from build123d import *

# Parameters (mm, degrees)
SKETCH3_R          = 4
CUT_EXTRUDE1_DEPTH = 14


with BuildPart() as part:
    # Sketch2 → Revolve1 (revolve)
    with BuildSketch(Plane(origin=(0, 0, 0), x_dir=(0, 0, -1), z_dir=(1, 0, 0)), mode=Mode.PRIVATE) as revolve1_sk:
        with BuildLine():
            Line((68.94, 0), (68.94, 32))
            Line((68.94, 32), (80, 32))
            Line((80, 32), (89.743935399, 25.177222982))
            ThreePointArc((89.743935399, 25.177222982), (86.850368108, 16), (89.743935399, 6.822777018))
            Line((89.743935399, 6.822777018), (80, 0))
            Line((80, 0), (68.94, 0))
        make_face()
    revolve(revolve1_sk.sketch.rotate(Axis((0, 24.773264932, 0), (0, -1, 0)), 180), axis=Axis((0, 24.773264932, 0), (0, -1, 0)))

    # Sketch3 → Cut-Extrude1 (cut)
    with BuildSketch(Plane(origin=(0, 0, 0), x_dir=(1, 0, 0), z_dir=(0, 1, 0))):
        with Locations((0, 68.94)):
            Circle(SKETCH3_R)
        with Locations((48.747941495, 48.747941495)):
            Circle(SKETCH3_R)
        with Locations((68.94, 0)):
            Circle(SKETCH3_R)
        with Locations((48.747941495, -48.747941495)):
            Circle(SKETCH3_R)
        with Locations((0, -68.94)):
            Circle(SKETCH3_R)
        with Locations((-48.747941495, -48.747941495)):
            Circle(SKETCH3_R)
        with Locations((-68.94, 0)):
            Circle(SKETCH3_R)
        with Locations((-48.747941495, 48.747941495)):
            Circle(SKETCH3_R)
    extrude(amount=CUT_EXTRUDE1_DEPTH, mode=Mode.SUBTRACT)


solid = part.part
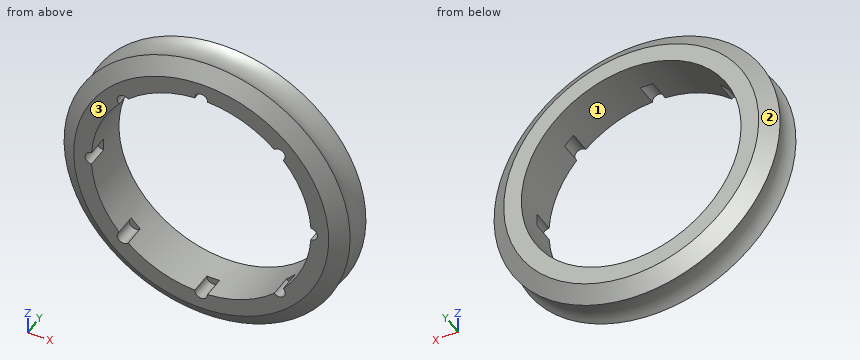
Verification items for the finished model (mm, model axes). Face numbers are marked on the shaded views. Round coordinates to 2 decimals unless told otherwise and drop trailing zeros. Loops run counter-clockwise (first coordinate to the right, second up) from the corner with the lowest first, then second, coordinate; pieces in that order, holes last. Notation, with made-up numbers: M 58.25,-19.5 L 88.25,-19.5 A15 cw 88.25,2.5 Z; hole C 81.5,75 d5. An arc over 180 degrees is marked long. Write each question's results on one line, items separated by ' | '.
1) Section check D-D on y = 17. Record the boundary of the cut face in (x, z).
Checks:
outline: C 0,0 d173.76; hole C 0,0 d137.88
2) Section check C-C on y = 28.5. Record the boundary of the cut face in (x, z).
Checks:
outline: C 0,0 d170; hole C 0,0 d137.88
3) Scan lines: L1, parallel to X at y = 15, z = 30.5; L2, parallel to X at y = 11, z = -62; L3, parallel to Z at x = -14.5, y = 6.5. Record each from-to range of solid material in increasing order. Write a range as from..to.
Checks:
L1: x = -81.35..-61.83, 61.83..81.35 | L2: x = -61.96..-30.15, 30.15..61.96 | L3: z = -88.1..-67.4, 67.4..88.1
4) Mould release check, pull along X, two halves, no side actions. Record for the marked faces 1, 2 and 3: released by +X, released by -X, zero draft, split by the parting line, or undercut.
Checks:
face 1: undercut | face 2: split by the parting line | face 3: zero draft
5) Gauge pin test, flat ends, axial feed: P1, Ø3.5, axis at x = -70, z = 1.5, coming from the -Y side; P2, Ø3, axis at x = 48.5, y = 26.5, coming from the +Z side; P3, Ø1, axis at x = 16.5, y = 5.5, coming from the +Z side. Record the tip position at first contact, or that the pin passes through.
Checks:
P1: stops at y = 14 | P2: stops at z = 75.96 | P3: stops at z = 87.02
6) Section check B-B on z = 0. Record the boundary of the cut face in (x, y), then the cut area to 3 significant figures.
Checks:
outline: M -89.74,6.82 L -80,0 L -72.94,0 L -72.94,14 L -68.94,14 L -68.94,32 L -80,32 L -89.74,25.18 A16 cw Z; M 68.94,14 L 72.94,14 L 72.94,0 L 80,0 L 89.74,6.82 A16 cw 89.74,25.18 L 80,32 L 68.94,32 Z | area: 1,010 mm2
7) Section check A-A on x = 0. Record the boundary of the cut face in (y, z), then the cut area to 3 significant figures.
Checks:
outline: M 0,-80 L 6.82,-89.74 A16 cw 25.18,-89.74 L 32,-80 L 32,-68.94 L 14,-68.94 L 14,-72.94 L 0,-72.94 Z; M 0,72.94 L 14,72.94 L 14,68.94 L 32,68.94 L 32,80 L 25.18,89.74 A16 cw 6.82,89.74 L 0,80 Z | area: 1,010 mm2
